Part print with two shaded views. Sizes in mm from the minimum x, y, z corner. Coordinates: 2 decimals unless noted, no trailing zeros. Loops run counter-clockwise (first coordinate to the right, second up) from the corner with the lowest first, then second, coordinate; pieces in that order, holes last. Notation, with made-up numbers: M 29.5,-25.75 L 72.5,-25.75 A33 ccw 72.5,3.25 Z; hole C 72.5,70 d11. An arc over 180 degrees is marked long. Write item = value, one per line. Start each with the question number.
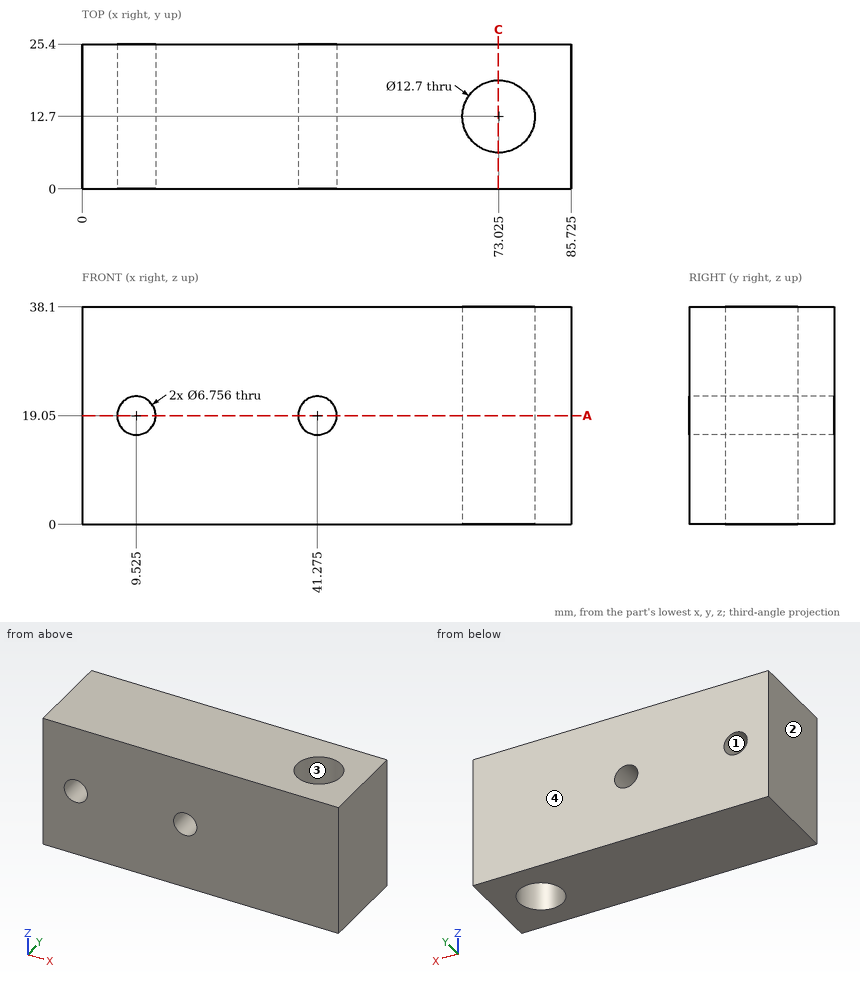
Item 1: Pull direction X, two halves, no side cores. Call the marked faces 1, 2, 3 and 4: +X half, -X half, draft (parallel to the pull), parting line (faces both ways), or undercut.
Item 2: Cut at C-C (x = 73). Give the cut face in (y, z), plus the area to 3 significant figures.
Item 3: Cut at A-A (z = 19.05). Give the number of separate pieces and of enclosed holes in the cut face, plus the area to 3 significant figures.
Item 4: Probe L1, parallel to X at y = 13, z = 19.05 (1 decimal); L2, parallel to X at y = 1, z = 19 (1 decimal); L3, parallel to X at y = 24, z = 18 (1 decimal). List the from-to ranges inside material, lowest first.
Reported:
q1.face_1 = undercut
q1.face_2 = -X half
q1.face_3 = undercut
q1.face_4 = draft
q2.outline = M 0,0 L 6.35,0 L 6.35,38.1 L 0,38.1 Z; M 19.05,0 L 25.4,0 L 25.4,38.1 L 19.05,38.1 Z
q2.area = 484 mm^2
q3.separate_pieces = 3
q3.enclosed_holes = 1
q3.area = 1,710 mm^2
q4.L1 = 0 to 6.1, 12.9 to 37.9, 44.7 to 66.7, 79.4 to 85.7
q4.L2 = 0 to 6.1, 12.9 to 37.9, 44.7 to 85.7
q4.L3 = 0 to 6.3, 12.7 to 38.1, 44.5 to 85.7
